from build123d import *

# Parameters (mm, degrees)
UBODY_SKETCH_R      = 5.5
UBODY_DEPTH         = 11.9
THREAD_SKETCH_W     = 2.415
THREAD_SKETCH_H     = 6.3
THREAD_CHAMFER_SIZE = 0.25
TUBE_START          = -13.3
TUBE_SKETCH_R       = 3.175
TUBE_DEPTH          = 13.3
TUBE_RADIUS_R       = 0.5
HEX_2_DEPTH         = 2
HEX_2_DRAFT         = -2
PORT_SKETCH_R       = 0.930158461
PORT_DEPTH          = 18.163624326


with BuildPart() as part:
    # Release_Sketch → Release (revolve)
    with BuildSketch(Plane.XY, mode=Mode.PRIVATE) as release_sk:
        with BuildLine():
            Line((0, 0), (-4.525, 0))
            ThreePointArc((-4.525, 0), (-4.878553391, -0.146446609), (-5.025, -0.5))
            Line((-5.025, -0.5), (-5.025, -1.5))
            Line((-5.025, -1.5), (-3.925, -1.5))
            Line((-3.925, -1.5), (-3.925, -2.4))
            Line((-3.925, -2.4), (0, -2.4))
            Line((0, -2.4), (0, 0))
        make_face()
    revolve(release_sk.sketch.rotate(Axis((0, 0, 0), (0, -1, 0)), 270), axis=Axis((0, 0, 0), (0, -1, 0)))

    # UBody_Sketch → UBody (add)
    with BuildSketch(Plane(origin=(0, -2.4, 0), x_dir=(-1, 0, 0), z_dir=(0, 1, 0))):
        with Locations(Location((0, 0, 0), (0, 0, 90))):
            Circle(UBODY_SKETCH_R)
    extrude(amount=-UBODY_DEPTH)

    # Thread_Sketch → Thread (revolve)
    with BuildSketch(Plane.XY, mode=Mode.PRIVATE) as thread_sk:
        with Locations((-1.2075, -17.45)):
            Rectangle(THREAD_SKETCH_W, THREAD_SKETCH_H)
    revolve(thread_sk.sketch.rotate(Axis((0, 0, 0), (0, -1, 0)), 270), axis=Axis((0, 0, 0), (0, -1, 0)))

    # Thread_Chamfer
    thread_chamfer_edges = [part.edges().sort_by_distance(p)[0] for p in [
        (0, -20.6, -2.415),
    ]]
    chamfer(thread_chamfer_edges, length=THREAD_CHAMFER_SIZE)

    # Tube_Sketch → Tube (cut)
    with BuildSketch(Plane(origin=(0, 0, 0), x_dir=(1, 0, 0), z_dir=(0, 1, 0)).offset(TUBE_START)):
        with Locations(Location((0, 0, 0), (0, 0, 270))):
            Circle(TUBE_SKETCH_R)
    extrude(amount=TUBE_DEPTH, mode=Mode.SUBTRACT)

    # Tube_Radius
    tube_radius_edges = [part.edges().sort_by_distance(p)[0] for p in [
        (0, 0, -3.175),
    ]]
    fillet(tube_radius_edges, radius=TUBE_RADIUS_R)


with BuildPart() as hex_2_tool:
    # Hex_Sketch → Hex 2 (with draft: the straight prism first)
    with BuildSketch(Plane(origin=(0, -13.3, 0), x_dir=(-1, 0, 0), z_dir=(0, 1, 0))):
        Polygon((-1.154700538, 0), (-0.577350269, -1), (0.577350269, -1), (1.154700538, 0), (0.577350269, 1), (-0.577350269, 1), align=None)
    extrude(amount=-HEX_2_DEPTH)
    # Hex 2: the draft: its side faces are tilted about the plane it starts from
    hex_2_sides = [hex_2_tool.faces().sort_by_distance(p)[0] for p in [
        (0.866025404, -14.3, -0.5),
        (0, -14.3, -1),
        (-0.866025404, -14.3, -0.5),
        (-0.866025404, -14.3, 0.5),
        (0, -14.3, 1),
        (0.866025404, -14.3, 0.5),
    ]]
    draft(hex_2_sides, Plane(origin=(0, -13.3, 0), x_dir=(-1, 0, 0), z_dir=(0, 1, 0)), HEX_2_DRAFT)


with BuildPart() as part_1:
    add(part.part)

    # Hex 2: cut by hex_2_tool
    add(hex_2_tool.part, mode=Mode.SUBTRACT)

    # Port_Sketch → Port (cut, through all)
    with BuildSketch(Plane(origin=(0, -15.3, 0), x_dir=(-1, 0, 0), z_dir=(0, 1, 0))):
        with Locations(Location((0, 0, 0), (0, 0, 90))):
            Circle(PORT_SKETCH_R)
    extrude(amount=-PORT_DEPTH, mode=Mode.SUBTRACT)


solid = part_1.part
Geometry: final body of the model. Coordinates: model frame, mm. A direction names the side the tool comes from. Give positions to 0.01 mm unless a question says otherwise; leave off trailing zeros. Loops run counter-clockwise (first coordinate to the right, second up) from the corner with the lowest first, then second, coordinate; pieces in that order, holes last. Notation, with made-up numbers: (-7.75, 9.5) -> (48.25, 9.5) arc R16 ccw to (48.25, 34.5) -> close; hole circle Ø5 at (-28, 32.5). An arc over 180 degrees is marked (long way). Put each result on its own line as item: value.
1. Cut plane B-B (y = -4.75). Return the cut outline in (x, z) (3 decimals), plus the area to 3 significant figures.
Taken from the geometry:
outline: circle Ø11 at (0, 0); hole circle Ø6.35 at (0, 0)
area: 63.4 mm2
2. Ray query, line 1 along X through (y, z) = (-5, 0) (3 decimals); line 2 along X through (y, z) = (-19.2, 0) (3 decimals); line 3 along Y through (x, z) = (3.75, 2.5). Return the intervals inside material, ascending. Write a range as [from, to].
Taken from the geometry:
line 1: x = [-5.5, -3.175], [3.175, 5.5]
line 2: x = [-2.415, -0.93], [0.93, 2.415]
line 3: y = [-14.3, -2.4], [-1.5, 0]
3. Pin query (flat end, axial travel): P1, Ø1.7, axis at x = 0, z = 0, coming from the -Y side; P2, Ø1.5, axis at x = 4.5, z = -3, coming from the +Y side; P3, Ø5, axis at x = 1, y = -8.5, coming from the -Z side; P4, Ø3, axis at y = -12.5, z = -3, coming from the +X side. Return the tip coordinate at first contact, or that it passes through.
Taken from the geometry:
P1: passes through
P2: stops at y = -0.02
P3: stops at z = -5.5
P4: stops at x = 5.29
4. Set-up query: faces 1 (the flat face through (-2.4, -14.3, 1.1)), 2 (the cylindrical face through (2.388, -1.956, -3.115)), 3 (the cylindrical face through (-0.91, -17.91, -0.2)), 4 (the flat face through (1, -13.3, -1)). Return all of +Z, -Z, +X, -X, +Y, -Y with unobstructed straight access to the full face (end or side cutting, diameter ignored); none if empty.
Taken from the geometry:
face 1: -Y
face 2: none
face 3: +Y, -Y
face 4: +Y
5. Pull-direction query (Z, two-part tool) for faces 5 (the flat face through (-4, 0, 0)), 6 (the cylindrical face through (-5.37, -8.27, -1.19)), 7 (the cylindrical face through (-1.93, -6.99, -2.52)); classes: released by +Z, released by -Z, zero draft, split by the parting line, or undercut.
Taken from the geometry:
face 5: zero draft
face 6: split by the parting line
face 7: undercut
6. Cut plane A-A (y = -2). Return the cut outline in (x, z) (3 decimals).
Taken from the geometry:
outline: circle Ø7.85 at (0, 0); hole circle Ø6.35 at (0, 0)
